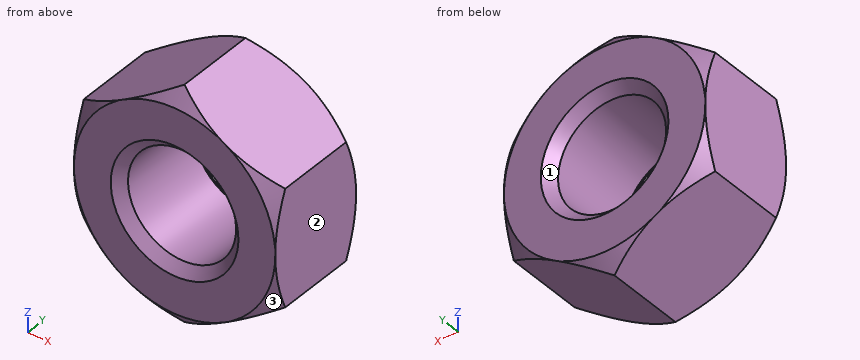
from build123d import *

# Parameters (mm, degrees)
BOSS_EXTRUDE1_DEPTH     = 5
SKETCH5_OUTSIDE_W       = 50.974
SKETCH5_OUTSIDE_H       = 53.914
SKETCH5_OUTSIDE_R       = 9.5
CUT_EXTRUDE1_DEPTH      = 10
CUT_EXTRUDE1_DRAFT      = -50
MIRROR1_COPY_1_SKETCH_W = 50.974
MIRROR1_COPY_1_SKETCH_H = 53.914
MIRROR1_COPY_1_SKETCH_R = 9.5
MIRROR1_COPY_1_DEPTH    = 10
MIRROR1_COPY_1_DRAFT    = -50


with BuildPart() as part:
    # Sketch1 → Boss-Extrude1 (new, symmetric)
    with BuildSketch(Plane(origin=(0, 0, 0), x_dir=(1, 0, 0), z_dir=(0, 1, 0))):
        Polygon((0, 10.969655115), (-9.5, 5.484827557), (-9.5, -5.484827557), (0, -10.969655115), (9.5, -5.484827557), (9.5, 5.484827557), align=None)
    extrude(amount=BOSS_EXTRUDE1_DEPTH, both=True)

    # Sketch4 → M12 Tapped Hole1 (revolve, cut)
    with BuildSketch(Plane(origin=(0, 5, 0), x_dir=(0, 0, 1), z_dir=(1, 0, 0))):
        Polygon((0, 0), (0, 10), (6.025, 10), (5.1, 9.075), (5.1, 0.925), (6.025, 0), align=None)
    revolve(axis=Axis((0, 11.35, 0), (0, -1, 0)), mode=Mode.SUBTRACT)


with BuildPart() as cut_extrude1_tool:
    # Sketch5 outside → Cut-Extrude1 (with draft: the straight prism first)
    with BuildSketch(Plane(origin=(0, 5, 0), x_dir=(1, 0, 0), z_dir=(0, 1, 0))):
        Rectangle(SKETCH5_OUTSIDE_W, SKETCH5_OUTSIDE_H)
        Circle(SKETCH5_OUTSIDE_R, mode=Mode.SUBTRACT)
    extrude(amount=-CUT_EXTRUDE1_DEPTH)
    # Cut-Extrude1: the draft: its side faces are tilted about the plane it starts from
    cut_extrude1_sides = [cut_extrude1_tool.faces().sort_by_distance(p)[0] for p in [
        (0, 0, 26.957),
        (25.487, 0, 0),
        (0, 0, -26.957),
        (-25.487, 0, 0),
        (-9.5, 0, 0),
    ]]
    draft(cut_extrude1_sides, Plane(origin=(0, 5, 0), x_dir=(1, 0, 0), z_dir=(0, 1, 0)), CUT_EXTRUDE1_DRAFT)


with BuildPart() as part_1:
    add(part.part)

    # Cut-Extrude1: cut by cut_extrude1_tool
    add(cut_extrude1_tool.part, mode=Mode.SUBTRACT)


with BuildPart() as mirror1_copy_1_tool:
    # Mirror1 copy 1 sketch → Mirror1 copy 1 (with draft: the straight prism first)
    with BuildSketch(Plane.XZ.offset(5)):
        Rectangle(MIRROR1_COPY_1_SKETCH_W, MIRROR1_COPY_1_SKETCH_H)
        Circle(MIRROR1_COPY_1_SKETCH_R, mode=Mode.SUBTRACT)
    extrude(amount=-MIRROR1_COPY_1_DEPTH)
    # Mirror1 copy 1: the draft: its side faces are tilted about the plane it starts from
    mirror1_copy_1_sides = [mirror1_copy_1_tool.faces().sort_by_distance(p)[0] for p in [
        (0, 0, 26.957),
        (25.487, 0, 0),
        (0, 0, -26.957),
        (-25.487, 0, 0),
        (-9.5, 0, 0),
    ]]
    draft(mirror1_copy_1_sides, Plane.XZ.offset(5), MIRROR1_COPY_1_DRAFT)


with BuildPart() as part_2:
    add(part_1.part)

    # Mirror1 copy 1: cut by mirror1_copy_1_tool
    add(mirror1_copy_1_tool.part, mode=Mode.SUBTRACT)


solid = part_2.part
Work out the finished part from the listing and answer in its coordinate system (mm). Face numbers are marked on the shaded views. Round coordinates to 2 decimals unless told otherwise and drop trailing zeros. Write each loop counter-clockwise with the first axis right and the second up, starting at its lowest first coordinate (ties: lowest second). Pieces come first, ordered by that corner, then holes. Notation, with made-up numbers: (10.25, 0.25) - (31.25, 0.25) arc R25 cw to (31.25, 35.25) - close; hole circle Ø4 at (30.25, 4.25). An arc over 180 degrees is marked (long way). Answer in a Markdown table with one row per item. Add a question column.
1. Given pin 1 (1 mm diameter, centred on x = -6, y = -2, fed in from +Z); pin 2 (3 mm diameter, centred on x = -6, y = -3, fed in from +Z); pin 3 (1.5 mm diameter, centred on x = -3.5, y = 2, fed in from +Z), each flat-ended and moving along its own axis, determine where each tip first touches the part or whether it passes through.
2. A cutting plane is placed at A-A, the plane y = 2.5. Determine the outline of the cut face in (x, z), and give its area (3 significant figures).
3. Find the intervals of material crossed by line 1 along X through (y, z) = (1.5, 0); line 2 along X through (y, z) = (-2.25, -3.5); line 3 along Z through (x, y) = (-0.25, 1.75), in increasing order. Write a range as from..to.
4. The mould has two halves that part along Z. Classify the marked faces 1, 2 and 3: +Z half, -Z half, draft (parallel to the pull), parting line (faces both ways), or undercut.
Worked out:
| question | item | result |
|---|---|---|
| 1 | pin 1 | z = 7.79 |
| 1 | pin 2 | z = 8.37 |
| 1 | pin 3 | z = 9.38 |
| 2 | outline | (-9.5, -5.48) - (0, -10.97) - (9.5, -5.48) - (9.5, 5.48) - (0, 10.97) - (-9.5, 5.48) - close; hole circle Ø10.2 at (0, 0) |
| 2 | area | 231 mm^2 |
| 3 | line 1 | -9.5..-5.1, 5.1..9.5 |
| 3 | line 2 | -9.5..-3.71, 3.71..9.5 |
| 3 | line 3 | -10.83..-5.09, 5.09..10.83 |
| 4 | face 1 | undercut |
| 4 | face 2 | draft |
| 4 | face 3 | -Z half |
